Source: CAD feature listing. Evaluate the final solid. Frame: model axes, mm. A direction names the side the tool comes from. Give positions to 0.01 mm unless a question says otherwise; leave off trailing zeros. Order: outer loops, then holes, each group sorted by start corner. A loop starts at its lowest first (then second) coordinate and runs counter-clockwise, first axis right, second up. Notation, with made-up numbers: (9, -14.75) -> (34, -14.75) arc R33 ccw to (34, 17.25) -> close; hole circle Ø3 at (79, 81). An arc over 180 degrees is marked (long way). Answer in a Markdown table with one row per item.
```python
from build123d import *

# Parameters (mm, degrees)
BOSS_EXTRUDE1_DEPTH = 19.05
BOSS_EXTRUDE2_START = 19.05
BOSS_EXTRUDE2_DEPTH = 4.7625
BOSS_EXTRUDE3_START = 19.05
BOSS_EXTRUDE3_DEPTH = 38.1
CUT_EXTRUDE1_DEPTH  = 16.875
SKETCH3_R           = 7.9375
BOSS_EXTRUDE5_DEPTH = 22.225
FILLET1_R           = 2.54


with BuildPart() as part:
    # Sketch1 → Boss-Extrude1 (new body)
    with BuildSketch(Plane(origin=(0, 0, 0), x_dir=(0, 0, -1), z_dir=(1, 0, 0))):
        with BuildLine():
            Line((0, 31.600913244), (0, 0))
            Line((0, 0), (98.425, 0))
            Line((98.425, 0), (98.425, 6.35))
            Line((98.425, 6.35), (120.65, 6.35))
            Line((120.65, 6.35), (120.65, 73.025))
            Line((120.65, 73.025), (133.35, 73.025))
            Line((133.35, 73.025), (133.35, 82.55))
            Line((133.35, 82.55), (107.95, 82.55))
            ThreePointArc((107.95, 82.55), (106.023410696, 82.353122997), (104.176464673, 81.770630688))
            Line((104.176464673, 81.770630688), (4.792887228, 38.888938818))
            ThreePointArc((4.792887228, 38.888938818), (1.305597176, 35.962308799), (0, 31.600913244))
        make_face()
        with BuildLine():
            ThreePointArc((41.696438991, 9.714502244), (22.962154899, 17.283644339), (30.531296995, 36.017928431))
            Line((30.531296995, 36.017928431), (62.679929002, 49.664213094))
            ThreePointArc((62.679929002, 49.664213094), (81.414213094, 42.095070998), (73.845070998, 23.360786906))
            Line((73.845070998, 23.360786906), (41.696438991, 9.714502244))
        make_face(mode=Mode.SUBTRACT)
        Polygon((98.425, 0), (0, 0), (0, -15.875), (120.65, -15.875), (120.65, 0), (120.65, 6.35), (98.425, 6.35), align=None)
        with BuildLine():
            Line((62.679929002, 49.664213094), (30.531296995, 36.017928431))
            ThreePointArc((30.531296995, 36.017928431), (22.962154899, 17.283644339), (41.696438991, 9.714502244))
            Line((41.696438991, 9.714502244), (73.845070998, 23.360786906))
            ThreePointArc((73.845070998, 23.360786906), (81.414213094, 42.095070998), (62.679929002, 49.664213094))
        make_face()
        with BuildLine():
            ThreePointArc((38.595010659, 17.021009518), (30.268662174, 20.385072672), (33.632725327, 28.711421157))
            Line((33.632725327, 28.711421157), (65.781357334, 42.357705819))
            ThreePointArc((65.781357334, 42.357705819), (74.107705819, 38.993642666), (70.743642666, 30.667294181))
            Line((70.743642666, 30.667294181), (38.595010659, 17.021009518))
        make_face(mode=Mode.SUBTRACT)
    extrude(amount=BOSS_EXTRUDE1_DEPTH)

    # Sketch1<3> → Boss-Extrude2 (add)
    with BuildSketch(Plane(origin=(0, 0, 0), x_dir=(0, 0, -1), z_dir=(1, 0, 0)).offset(BOSS_EXTRUDE2_START)):
        with BuildLine():
            Line((41.696438991, 9.714502244), (73.845070998, 23.360786906))
            ThreePointArc((73.845070998, 23.360786906), (81.414213094, 42.095070998), (62.679929002, 49.664213094))
            Line((62.679929002, 49.664213094), (30.531296995, 36.017928431))
            ThreePointArc((30.531296995, 36.017928431), (22.962154899, 17.283644339), (41.696438991, 9.714502244))
        make_face()
        with BuildLine():
            ThreePointArc((33.632725327, 28.711421157), (30.268662174, 20.385072672), (38.595010659, 17.021009518))
            Line((38.595010659, 17.021009518), (70.743642666, 30.667294181))
            ThreePointArc((70.743642666, 30.667294181), (74.107705819, 38.993642666), (65.781357334, 42.357705819))
            Line((65.781357334, 42.357705819), (33.632725327, 28.711421157))
        make_face(mode=Mode.SUBTRACT)
    extrude(amount=BOSS_EXTRUDE2_DEPTH)

    # Sketch1<4> → Boss-Extrude3 (add)
    with BuildSketch(Plane(origin=(0, 0, 0), x_dir=(0, 0, -1), z_dir=(1, 0, 0)).offset(BOSS_EXTRUDE3_START)):
        Polygon((98.425, 0), (0, 0), (0, -15.875), (120.65, -15.875), (120.65, 0), (120.65, 6.35), (98.425, 6.35), align=None)
    extrude(amount=BOSS_EXTRUDE3_DEPTH)

    # Sketch2 → Cut-Extrude1 (cut, through all)
    with BuildSketch(Plane(origin=(0, 0, 0), x_dir=(1, 0, 0), z_dir=(0, 1, 0))):
        Polygon((19.05, 0), (57.15, 98.425), (57.15, 0), align=None)
    extrude(amount=-CUT_EXTRUDE1_DEPTH, mode=Mode.SUBTRACT)

    # Sketch3 → Boss-Extrude5 (add)
    with BuildSketch(Plane(origin=(0, 0, -120.65), x_dir=(-1, 0, 0), z_dir=(0, 0, -1))):
        with BuildLine():
            Line((-19.05, 0), (-47.625, 0))
            ThreePointArc((-47.625, 0), (-66.675, 19.05), (-47.625, 38.1))
            Line((-47.625, 38.1), (-19.05, 38.1))
            Line((-19.05, 38.1), (-19.05, 0))
        make_face()
        with Locations((-47.625, 19.05)):
            Circle(SKETCH3_R, mode=Mode.SUBTRACT)
    extrude(amount=-BOSS_EXTRUDE5_DEPTH)

    # Fillet1
    fillet1_edges = [part.edges().sort_by_distance(p)[0] for p in [
        (57.15, 2.552216058, -109.5375),
    ]]
    fillet(fillet1_edges, radius=FILLET1_R)


solid = part.part
```
(1) Pull-direction query (Y, two-part tool) for faces 6 (the flat face through (9, 82.55, -121)), 7 (the cylindrical face through (11.74, 38.865, -74.161)), 8 (the flat face through (9, 73.025, -127)), 9 (the cylindrical face through (40.293, 16.01, -109.693)); classes: +Y half, -Y half, draft (parallel to the pull), parting line (faces both ways), or undercut.
A:
| item | result |
|---|---|
| face 6 | +Y half |
| face 7 | undercut |
| face 8 | -Y half |
| face 9 | undercut |
(2) Section query C-C (y = 19.05). Give the number of separate pieces and of enclosed holes in the cut face, plus the area to 3 significant figures.
A:
| item | result |
|---|---|
| separate pieces | 3 |
| enclosed holes | 0 |
| area | 2,910 mm^2 |
(3) First-contact query: pin 1 Ø10 at (y, z) = (34, -80) entering from +X; pin 2 Ø12 at (x, z) = (43.5, -77.5) entering from +Y; pin 3 Ø8 at (y, z) = (59, -106.5) entering from +X. Flat tips, straight axial feed; report the tip coordinate or a pass-through.
A:
| item | result |
|---|---|
| pin 1 | stops at x = 23.81 |
| pin 2 | stops at y = 0 |
| pin 3 | stops at x = 19.05 |
(4) Access query for faces 1 (the flat face through (19.05, 51, -66)), 2 (the flat face through (23.812, 25, -59)), 3 (the flat face through (11.74, 23.749, -54.444)), 4 (the flat face through (57.15, -7, -109)), 5 (the flat face through (9, 78, -133.35)). Directions: +Z, -Z, +X, -X, +Y, -Y. A direction counts if a zero-diameter tool reaches every point of the face in a straight line with its end or side. Return the directions, or none.
A:
| item | result |
|---|---|
| face 1 | +X |
| face 2 | +Z, +X, +Y |
| face 3 | +X, -X |
| face 4 | +Z, -Z, +X, -Y |
| face 5 | -Z, +X, -X, +Y, -Y |
(5) Ray query, probe 1 along X at (y, z) = (19, -113); probe 2 along Y at (x, z) = (23, -68.5) (3 decimals); probe 3 along X at (y, z) = (58, -51). Return the intervals inside material, ascending.
A:
| item | result |
|---|---|
| probe 1 | x = 0 to 39.69, 55.56 to 66.67 |
| probe 2 | y = -15.875 to 0, 21.092 to 29.715, 42.858 to 50.798 |
| probe 3 | x = 0 to 19.05 |
(6) Section query D-D (x = 31). Return the cut outline in (y, z) (3 decimals), plus the area to 3 significant figures.
A:
| item | result |
|---|---|
| outline | (-15.875, -120.65) -> (38.1, -120.65) -> (38.1, -98.425) -> (0, -98.425) -> (0, -30.871) -> (-15.875, -30.871) -> close |
| area | 2,270 mm^2 |
